For this review, take the finished solid that the model builds, in its own axes (mm). A direction names the side the tool comes from. Coordinates: 2 decimals unless noted, no trailing zeros. Loops run counter-clockwise (first coordinate to the right, second up) from the corner with the lowest first, then second, coordinate; pieces in that order, holes last.
1. Take a section at B-B, the plane y = 41.5. State the section outline as (x, z) points, then the cut area to 3 significant figures.
2. Clearance check with flat-ended pins moving along their axes: P1, Ø6, axis at x = 43, y = 51, coming from the -Z side; P2, Ø1.5, axis at x = 197.5, y = 37, coming from the +Z side; P3, Ø10, axis at x = -6, z = 88.5, coming from the +Y side. State where each tip first meets the part, or that it passes through.
3. Take a section at C-C, the plane z = 0. State the section outline as (x, y) points, then the cut area to 3 significant figures.
4. Mouldability with a two-part tool opening along Z and no side actions: class faces 1 (the face through (-3, 17.462, -15)), 2 (the face through (243.07, 63.19, -72.35)), 3 (the face through (-3, 9, -172.212)) as pulls with the +Z half, pulls with the -Z half, needs draft (parallel to the pull), parting line crosses it, or undercut.
5. Take a section at A-A, the plane x = 0. State the section outline as (y, z) points, then the cut area to 3 significant figures.
6. Take a section at D-D, the plane x = 146. State the section outline as (y, z) points, then the cut area to 3 significant figures.
7. To check wall thickness, follow probe 1 along X at (y, z) = (5, 0); probe 2 along Z at (x, y) = (0, 9); probe 3 along Z at (x, y) = (-25, 59). State the ranges of each line that lie inside material, in increasing order.
8. Machinability: for faces 4 (the face through (248.412, 14, 2)), 5 (the face through (-3, 68.262, -72)), 6 (the face through (-3, 17.462, 126)), 7 (the face through (-3, 43, -63.5)), 8 (the face through (-3, 17.462, -127)), which of the approach directions +Z, -Z, +X, -X, +Y, -Y give a long, thin tool a straight path to every point of the face, cutting with its end or side? Answer none if there is none.
```python
from build123d import *

# Parameters (mm, degrees)
SKETCH1_W           = 496.824
SKETCH1_H           = 344.424
BOSS_EXTRUDE1_DEPTH = 17.4625
CUT_EXTRUDE1_REACH  = 19.462
SKETCH3_R           = 6.76275
SKETCH5_W           = 496.824
SKETCH5_H           = 17.4625
BOSS_EXTRUDE2_DEPTH = 50.8
FILLET2_R           = 17.78


with BuildPart() as part:
    # Sketch1 → Boss-Extrude1 (new body)
    with BuildSketch(Plane(origin=(0, 0, 0), x_dir=(1, 0, 0), z_dir=(0, 1, 0))):
        Rectangle(SKETCH1_W, SKETCH1_H)
    extrude(amount=BOSS_EXTRUDE1_DEPTH)

    # Sketch3 → Cut-Extrude1 (cut, up to next)
    with BuildSketch(Plane(origin=(0, 17.4625, 0), x_dir=(1, 0, 0), z_dir=(0, 1, 0)), mode=Mode.PRIVATE) as cut_extrude1_sk1:
        Circle(SKETCH3_R)
    cut_extrude1_tool1 = extrude(cut_extrude1_sk1.sketch, amount=-CUT_EXTRUDE1_REACH, mode=Mode.PRIVATE) & part.part
    add(cut_extrude1_tool1.solids().sort_by_distance((0, 17.4625, 0))[0], mode=Mode.SUBTRACT)

    # Sketch5 → Boss-Extrude2 (add)
    with BuildSketch(Plane(origin=(0, 17.4625, 0), x_dir=(1, 0, 0), z_dir=(0, 1, 0))):
        with Locations((0, 72.23125)):
            Rectangle(SKETCH5_W, SKETCH5_H)
    boss_extrude2 = extrude(amount=BOSS_EXTRUDE2_DEPTH)

    # Mirror1: Boss-Extrude2 across plane
    add(boss_extrude2.mirror(Plane.XY))

    # Fillet2
    fillet2_edges = [part.edges().sort_by_distance(p)[0] for p in [
        (-248.412, 68.2625, -72.23125),
        (248.412, 68.2625, -72.23125),
        (-248.412, 68.2625, 72.23125),
        (248.412, 68.2625, 72.23125),
    ]]
    fillet(fillet2_edges, radius=FILLET2_R)


solid = part.part
```
Results list:
1. outline: (-248.41, -80.96) - (248.41, -80.96) - (248.41, -63.5) - (-248.41, -63.5) - close; (-248.41, 63.5) - (248.41, 63.5) - (248.41, 80.96) - (-248.41, 80.96) - close
1. area: 17,400 mm2
2. P1: stops at z = -80.96
2. P2: stops at z = 80.96
2. P3: stops at y = 17.46
3. outline: (-248.41, 0) - (-6.76, 0) - (-6.76, 17.46) - (-248.41, 17.46) - close; (6.76, 0) - (248.41, 0) - (248.41, 17.46) - (6.76, 17.46) - close
3. area: 8,440 mm2
4. face 1: undercut
4. face 2: needs draft
4. face 3: pulls with the -Z half
5. outline: (0, -172.21) - (17.46, -172.21) - (17.46, -80.96) - (68.26, -80.96) - (68.26, -63.5) - (17.46, -63.5) - (17.46, -6.76) - (0, -6.76) - close; (0, 6.76) - (17.46, 6.76) - (17.46, 63.5) - (68.26, 63.5) - (68.26, 80.96) - (17.46, 80.96) - (17.46, 172.21) - (0, 172.21) - close
5. area: 7,550 mm2
6. outline: (0, -172.21) - (17.46, -172.21) - (17.46, -80.96) - (68.26, -80.96) - (68.26, -63.5) - (17.46, -63.5) - (17.46, 63.5) - (68.26, 63.5) - (68.26, 80.96) - (17.46, 80.96) - (17.46, 172.21) - (0, 172.21) - close
6. area: 7,790 mm2
7. probe 1: x = -248.41 to -6.76, 6.76 to 248.41
7. probe 2: z = -172.21 to -6.76, 6.76 to 172.21
7. probe 3: z = -80.96 to -63.5, 63.5 to 80.96
8. face 4: +Z, -Z, +X, +Y, -Y
8. face 5: +Z, -Z, +X, -X, +Y
8. face 6: +Z, +X, -X, +Y
8. face 7: +X, -X, +Y
8. face 8: -Z, +X, -X, +Y
